The listing builds one solid part. Answer for the finished solid, in the listing's coordinates (mm). Face numbers are marked on the shaded views. A direction names the side the tool comes from. Round coordinates to 2 decimals unless told otherwise and drop trailing zeros. Loops run counter-clockwise (first coordinate to the right, second up) from the corner with the lowest first, then second, coordinate; pieces in that order, holes last. Notation, with made-up numbers: M 17,32.5 L 56,32.5 A21 cw 56,58.5 Z; hole C 31.25,-12.75 d1. An arc over 180 degrees is marked long. Put each result on its own line as item: value. Start each with the question number.
(1) Section A-A, the plane x = 19 is taken. Determine the outline of the cut face in (y, z).
(2) Straight lines are drawn through the part: line 1 (Y direction, x = 9.5, z = -7.5); line 2 (Z direction, x = 23.5, y = 9.25); line 3 (Y direction, x = 34, z = 4). For each, find the intervals that lie inside material, in ascending order.
(3) Section B-B, the plane x = 25.5 is taken. Determine the outline of the cut face in (y, z).
(4) Flat-ended cylindrical pins translate along their axes: P1, Ø4, axis at x = 26.5, z = -6.5, coming from the -Y side; P2, Ø2, axis at x = 25.5, z = -3.5, coming from the +Y side; P3, Ø5, axis at x = 16.5, z = 10, coming from the -Y side. Find the tip coordinate at first contact, or state that the pin passes through.
(5) Determine the mould class of the marked faces 3, 4 and 5 for opening direction X: released by +X, released by -X, zero draft, split by the parting line, or undercut.
(6) Which of the six approach directions +Z, -Z, +X, -X, +Y, -Y give full straight-line access (tool end or side, diameter ignored) to the marked faces 1 and 2?
Autodesk Inventor part; units mm, degrees
ref_plane "YZ Plane" through (0, 0, 0) normal (1, 0, 0) x (0, 1, 0)
ref_plane "XZ Plane" through (0, 0, 0) normal (0, 1, 0) x (-1, 0, 0)
ref_plane "XY Plane" through (0, 0, 0) normal (0, 0, 1) x (1, 0, 0)
sketch "Sketch1" plane through (0, 0, 0) normal (0, 0, 1) x (1, 0, 0)
  line L0 (0, 0) -> (6.6144, 0) construction
  line L1 (0, 0) -> (0, 4.75) construction
  line L2 (0, 4.75) -> (8, 4.3864)
  line L3 (6.6144, 0) -> (16.6144, 0) construction
  line L4 (16.6144, 0) -> (16.6144, 11.25) construction
  line L5 (16.6144, 0) -> (36.6144, 0) construction
  line L6 (36.6144, 0) -> (36.6144, 11) construction
  line L7 (36.6144, 11) -> (16.6144, 11.25)
  line L8 (0, 4.75) -> (0, 6.75)
  line L9 (0, 4.75) -> (2, 4.75) construction
  line L10 (0, 6.75) -> (16.6144, 11.25)
  line L11 (8, 4.3864) -> (16.6144, 10.05)
  line L12 (16.6144, 10.05) -> (36.6144, 9.7999)
  line L13 (36.6144, 9.7999) -> (36.6144, 11)
  line L14 (0, 0) -> (3.3, 0) construction
  line L15 (3.3, 0) -> (3.3, 4.6) construction
  dimension "d2" = 4.75
  dimension "d3" = 11.25
  dimension "d4" = 20
  dimension "d5" = 11
  dimension "d6" = 2
  dimension "d7" = 90
  dimension "d8" = 1.2
  dimension "d9" = 1.2
  dimension "d10" = 10
  dimension "d24" = 177.397
  dimension "d25" = 8
  dimension "d26" = 3.3
  dimension "d27" = 4.6
  dimension "d28" = 6.6144
revolve "Revolution1" add sketch "Sketch1" angle 360 about axis through (6.6144, 0, 0) along (1, 0, 0)
sketch "Sketch2" plane through (0, 0, 0) normal (-1, 0, 0) x (0, 0, 1)
  circle A0 centre (0, 0) radius 6.75
  line L0 (0, -6.75) -> (0, -11.25) construction
  circle A1 centre (0, 0) radius 11.25
  line L1 (1.633, -6.5495) -> (2.7216, -10.9158)
  line L2 (-1.633, -6.5495) -> (-2.7216, -10.9158)
  point P0 (-1.633, -6.5495)
  dimension "d12" = 14
extrude "Extrusion1" [suppressed]
chamfer "Chamfer1" [suppressed]
pattern_circular "Circular Pattern1" [suppressed]
chamfer "Chamfer2" distance 0.7 angle 45 1 edges at (0, -4.75, 0)
sketch "Sketch3" plane through (0, 0, 0) normal (-1, 0, 0) x (0, 0, 1)
  line L0 (-6.9282, -12) -> (-13.8564, 0)
  line L1 (-13.8564, 0) -> (-6.9282, 12)
  line L2 (-6.9282, 12) -> (6.9282, 12)
  line L3 (6.9282, 12) -> (13.8564, 0)
  line L4 (13.8564, 0) -> (6.9282, -12)
  line L5 (6.9282, -12) -> (-6.9282, -12)
  circle A0 centre (0, 0) radius 6.75
  point P0 (0, -12)
  dimension "d32" = 24
extrude "Extrusion2" add sketch "Sketch3" against normal blind 10
fillet "Fillet1" radius 2 6 edges at (5, 12, 6.9282) (5, 12, -6.9282) (5, 0, -13.8564) (5, -12, -6.9282) (5, -12, 6.9282) (5, 0, 13.8564)
equation "\"Tol\" = 0"
properties part number "PneumaticAdaptor"
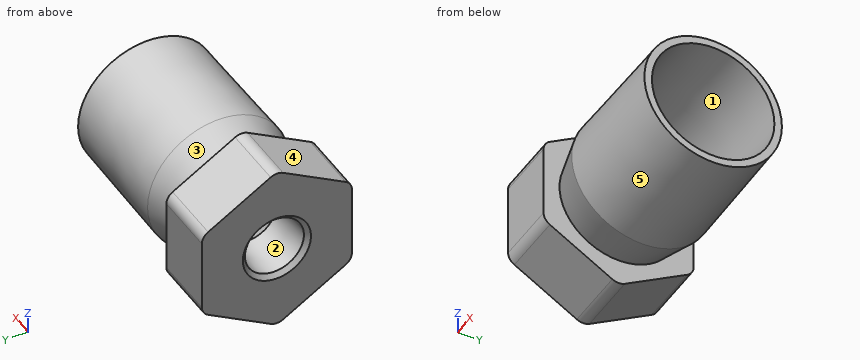
Recorded:
1. outline: C 0,0 d22.44; hole C 0,0 d20.04
2. line 1: y = -11.01 to 11.01
2. line 2: z = -6.25 to -3.7, 3.7 to 6.25
2. line 3: y = -10.28 to -8.98, 8.98 to 10.28
3. outline: C 0,0 d22.28; hole C 0,0 d19.88
4. P1: stops at y = -10.18
4. P2: stops at y = 10.86
4. P3: stops at y = -8.38
5. face 3: undercut
5. face 4: zero draft
5. face 5: released by +X
6. face 1: none
6. face 2: -X
